For this review, take the finished solid that the model builds, in its own axes (mm). Round coordinates to 2 decimals unless told otherwise and drop trailing zeros. Write each loop counter-clockwise with the first axis right and the second up, starting at its lowest first coordinate (ties: lowest second). Pieces come first, ordered by that corner, then holes.
from build123d import *

# Parameters (mm, degrees)
SKETCH1_R                = 19.05
BOSS_EXTRUDE1_DEPTH      = 100
BOSS_EXTRUDE2_REACH      = 105.565
BOSS_EXTRUDE2_END_RADIUS = 5
SKETCH3_R                = 2.5


with BuildPart() as part:
    # Sketch1 → Boss-Extrude1 (new body)
    with BuildSketch(Plane(origin=(0, 70, 0), x_dir=(-1, 0, 0), z_dir=(0, 1, 0))):
        with Locations(Location((0, 0, 0), (0, 0, 90))):
            Circle(SKETCH1_R)
    extrude(amount=BOSS_EXTRUDE1_DEPTH)



with BuildPart() as body_2:
    # Sketch2 → Revolve1 (revolve)
    with BuildSketch(Plane(origin=(0, 0, 0), x_dir=(1, 0, 0), z_dir=(0, 1, 0))):
        with BuildLine():
            Line((-5, 0), (5, 0))
            ThreePointArc((5, 0), (0, -5), (-5, 0))
        make_face()
    revolve(axis=Axis((-5, 0, 0), (1, 0, 0)))


with BuildPart() as part_1:
    add(part.part)

    add(body_2.part)  # Boss-Extrude2 merges body 2
    # Boss-Extrude2: up to this sphere (the profile starts outside it)
    boss_extrude2_end = Location((0, 0, 0)) * Sphere(BOSS_EXTRUDE2_END_RADIUS, mode=Mode.PRIVATE)
    # Sketch3 → Boss-Extrude2 (add, up to the surface)
    with BuildSketch(Plane.XZ.offset(-70), mode=Mode.PRIVATE) as boss_extrude2_sk1:
        with Locations(Location((0, 0, 0), (0, 0, 90))):
            Circle(SKETCH3_R)
    boss_extrude2_tool1 = extrude(boss_extrude2_sk1.sketch, amount=BOSS_EXTRUDE2_REACH, mode=Mode.PRIVATE) - boss_extrude2_end
    add(boss_extrude2_tool1.solids().sort_by_distance((0, 70, 0))[0])


solid = part_1.part
(1) For line 1 along Y through (x, z) = (6.5, 17.5); line 2 along Z through (x, y) = (-8, 161); line 3 along X through (y, z) = (155.5, -10), list the stretches that pass through material, from the lowest coordinate up.
Geometry check:
line 1: y = 70 to 170
line 2: z = -17.29 to 17.29
line 3: x = -16.21 to 16.21
(2) We need section D-D, the plane y = 87. Give the boundary of the cut face in (x, z), and give its area (3 significant figures).
Geometry check:
outline: circle Ø38.1 at (0, 0)
area: 1,140 mm2
(3) We need section C-C, the plane y = 53.5. Give the boundary of the cut face in (x, z).
Geometry check:
outline: circle Ø5 at (0, 0)
(4) Mouldability with a two-part tool opening along Y and no side actions: class faces 1 (the face through (0, 170, 0)), 2 (the face through (-11.59, 119.3, -15.12)), 3 (the face through (2.44, 37.62, -0.54)) as pulls with the +Y half, pulls with the -Y half, needs draft (parallel to the pull), parting line crosses it, or undercut.
Geometry check:
face 1: pulls with the +Y half
face 2: needs draft
face 3: undercut
(5) We need section A-A, the plane x = 0. Give the boundary of the cut face in (y, z).
Geometry check:
outline: (4.33, -2.5) - (70, -2.5) - (70, -19.05) - (170, -19.05) - (170, 19.05) - (70, 19.05) - (70, 2.5) - (4.33, 2.5) arc R5 ccw (long way) to start
(6) We need section B-B, the plane z = 0. Give the boundary of the cut face in (x, y).
Geometry check:
outline: (-19.05, 70) - (-2.5, 70) - (-2.5, 4.33) arc R5 ccw (long way) to (2.5, 4.33) - (2.5, 70) - (19.05, 70) - (19.05, 170) - (-19.05, 170) - close
(7) For pin 1 Ø12 at (y, z) = (81.5, -0.5) entering from +X; pin 2 Ø2 at (x, y) = (9, 102) entering from +Z; pin 3 Ø5 at (y, z) = (91, 4.5) entering from +X; pin 4 Ø5 at (x, y) = (14, 66.5) entering from +Z, all flat-tipped, find the tip position at first contact; note any pin that passes through.
Geometry check:
pin 1: stops at x = 19.05
pin 2: stops at z = 17.29
pin 3: stops at x = 18.94
pin 4: passes through
